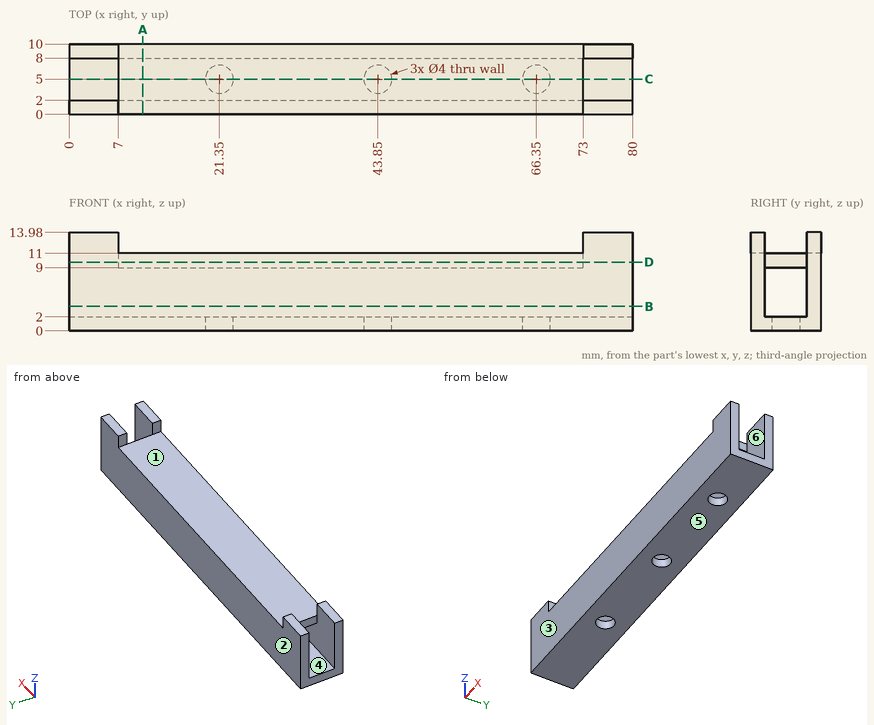
The figure shows three views and two pictorial views of one solid part (mm, origin at its lowest corner). Answer the questions. A direction names the side the tool comes from. Give positions to 0.01 mm unless a question says otherwise; leave off trailing zeros. Write each loop counter-clockwise with the first axis right and the second up, starting at its lowest first coordinate (ties: lowest second). Pieces come first, ordered by that corner, then holes.
Q1. The part is cut by section C-C on y = 5. Give the vertices of the cut face in (x, z).
Answer:
outline: (0, 0) - (19.35, 0) - (19.35, 2) - (0, 2) - close; (7, 9) - (73, 9) - (73, 11) - (7, 11) - close; (23.35, 0) - (41.85, 0) - (41.85, 2) - (23.35, 2) - close; (45.85, 0) - (64.35, 0) - (64.35, 2) - (45.85, 2) - close; (68.35, 0) - (80, 0) - (80, 2) - (68.35, 2) - close
Q2. The part is cut by section B-B on z = 3.5. Give the vertices of the cut face in (x, y), and give its area (3 significant figures).
Answer:
outline: (0, 0) - (80, 0) - (80, 2) - (0, 2) - close; (0, 8) - (80, 8) - (80, 10) - (0, 10) - close
area: 320 mm2
Q3. Straight lines are drawn through the part: L1, parallel to Y at x = 59, z = 6.25; L2, parallel to Z at x = 8, y = 3; L3, parallel to Z at x = 22, y = 6.5. For each, find the intervals that lie inside material, in ascending order.
Answer:
L1: y = 0 to 2, 8 to 10
L2: z = 0 to 2, 9 to 11
L3: z = 9 to 11
Q4. A tool of negligible diameter and unlimited length cuts with its end or side. For the marked faces 1 and 2, from which of +Z, -Z, +X, -X, +Y, -Y can it reach the whole face along a straight path? Write none if from no direction.
Answer:
face 1: +Z, +Y, -Y
face 2: +Z, -Z, +X, -X, +Y
Q5. The part is cut by section A-A on x = 10.5. Give the vertices of the cut face in (y, z).
Answer:
outline: (0, 0) - (10, 0) - (10, 11) - (0, 11) - close; hole (2, 2) - (8, 2) - (8, 9) - (2, 9) - close
Q6. For a pull along Y with two mould halves and no side action, classify the marked faces 3, 4, 5 and 6 as released by +Y, released by -Y, zero draft, split by the parting line, or undercut.
Answer:
face 3: released by -Y
face 4: undercut
face 5: zero draft
face 6: undercut
Q7. The part is cut by section D-D on z = 9.75. Give the vertices of the cut face in (x, y).
Answer:
outline: (0, 0) - (80, 0) - (80, 2) - (73, 2) - (73, 8) - (80, 8) - (80, 10) - (0, 10) - (0, 8) - (7, 8) - (7, 2) - (0, 2) - close
Q8. Given pin 1 (2 mm diameter, centred on y = 6, z = 10.5, fed in from -X); pin 2 (6 mm diameter, centred on x = 45, y = 1.5, fed in from +Z); pin 3 (1.6 mm diameter, centred on y = 4.5, z = 10, fed in from +X), each flat-ended and moving along its own axis, determine where each tip first touches the part or whether it passes through.
Answer:
pin 1: stops at x = 7
pin 2: stops at z = 11
pin 3: stops at x = 73
